Work out the finished part from the listing and answer in its coordinate system (mm). A direction names the side the tool comes from. Give positions to 0.01 mm unless a question says otherwise; leave off trailing zeros. Loops run counter-clockwise (first coordinate to the right, second up) from the corner with the lowest first, then second, coordinate; pieces in that order, holes last. Notation, with made-up numbers: M 87.5,71 L 145.5,71 A21 ccw 145.5,79 Z; hole C -0.5,-17 d4. An arc over 180 degrees is marked long. Answer as a JSON object with one key per item and string values. Group by question number.
```python
from build123d import *

# Parameters (mm, degrees)
SALIENTE_EXTRUIR1_DEPTH = 3
SALIENTE_EXTRUIR2_DEPTH = 9.75
CROQUIS6_R              = 1.625
CORTAR_EXTRUIR1_DEPTH   = 5
CORTAR_EXTRUIR2_DEPTH   = 2
CORTAR_EXTRUIR4_DEPTH   = 10
CROQUIS10_R             = 1.625
SALIENTE_EXTRUIR3_DEPTH = 2
CROQUIS12_R             = 1.625
CORTAR_EXTRUIR5_DEPTH   = 5
CORTAR_EXTRUIR6_DEPTH   = 2
CROQUIS14_R             = 1.625
CORTAR_EXTRUIR7_DEPTH   = 4
CORTAR_EXTRUIR8_DEPTH   = 2
CROQUIS17_R             = 1.625
CORTAR_EXTRUIR9_DEPTH   = 4
CORTAR_EXTRUIR10_DEPTH  = 2


with BuildPart() as part:
    # Croquis1 → Saliente-Extruir1 (new body)
    with BuildSketch(Plane.XY):
        with BuildLine():
            Line((0, 0.68070798), (0, 0))
            Line((0, 0), (72.78319995, 0))
            Line((72.78319995, 0), (55.699999998, 14.642073221))
            Line((55.699999998, 14.642073221), (46.67593732, 50.511923567))
            Line((46.67593732, 50.511923567), (-35.562657036, 50.511923567))
            Line((-35.562657036, 50.511923567), (-35.562657036, 38.25))
            Line((-35.562657036, 38.25), (-8.913300435, 38.25))
            Line((-8.913300435, 38.25), (-3.562657036, 35.25))
            ThreePointArc((-3.562657036, 35.25), (6.381456753, 18.806597842), (0, 0.68070798))
        make_face()
    extrude(amount=-SALIENTE_EXTRUIR1_DEPTH)

    # Croquis5 → Saliente-Extruir2 (add)
    with BuildSketch(Plane(origin=(0, 0, -3), x_dir=(-1, 0, 0), z_dir=(0, 0, -1))):
        with BuildLine():
            Line((-51.238983488, 11.880365447), (-59.266443595, 5))
            Line((-59.266443595, 5), (-3.339079606, 5))
            ThreePointArc((-3.339079606, 5), (-1.801031086, 2.738703104), (0, 0.68070798))
            Line((0, 0.68070798), (0, 0))
            Line((0, 0), (-72.78319995, 0))
            Line((-72.78319995, 0), (-55.699999998, 14.642073221))
            Line((-55.699999998, 14.642073221), (-46.67593732, 50.511923567))
            Line((-46.67593732, 50.511923567), (35.562657036, 50.511923567))
            Line((35.562657036, 50.511923567), (35.562657036, 38.25))
            Line((35.562657036, 38.25), (31.562657036, 38.25))
            Line((31.562657036, 38.25), (31.562657036, 46.511923567))
            Line((31.562657036, 46.511923567), (-42.526447804, 46.511923567))
            Line((-42.526447804, 46.511923567), (-51.238983488, 11.880365447))
        make_face()
    extrude(amount=SALIENTE_EXTRUIR2_DEPTH)

    # Croquis6 → Cortar-Extruir1 (cut)
    with BuildSketch(Plane.XZ):
        with Locations((6.999999998, -7)):
            Circle(CROQUIS6_R)
        with Locations((52.78319995, -7)):
            Circle(CROQUIS6_R)
    extrude(amount=-CORTAR_EXTRUIR1_DEPTH, mode=Mode.SUBTRACT)

    # Croquis8 → Cortar-Extruir2 (cut)
    with BuildSketch(Plane(origin=(0, 5, 0), x_dir=(1, 0, 0), z_dir=(0, 1, 0))):
        Polygon((3.819999998, 7), (5.409999998, 4.246039216), (8.589999998, 4.246039216), (10.179999998, 7), (8.589999998, 9.753960784), (5.409999998, 9.753960784), align=None)
        Polygon((49.60319995, 7), (51.19319995, 4.246039216), (54.37319995, 4.246039216), (55.96319995, 7), (54.37319995, 9.753960784), (51.19319995, 9.753960784), align=None)
    extrude(amount=-CORTAR_EXTRUIR2_DEPTH, mode=Mode.SUBTRACT)

    # Croquis9 → Cortar-Extruir4 (cut)
    with BuildSketch(Plane(origin=(30.824200619, 35.963211942, 0), x_dir=(0.759271307, -0.650774217, 0), z_dir=(0.650774217, 0.759271307, 0))):
        Polygon((50.442195378, 6.375), (48.852195378, 9.128960784), (45.672195378, 9.128960784), (44.082195378, 6.375), (45.672195378, 3.621039216), (48.852195378, 3.621039216), align=None)
    extrude(amount=-CORTAR_EXTRUIR4_DEPTH, mode=Mode.SUBTRACT)

    # Croquis10 → Saliente-Extruir3 (add)
    with BuildSketch(Plane(origin=(30.824200619, 35.963211942, 0), x_dir=(0.759271307, -0.650774217, 0), z_dir=(0.650774217, 0.759271307, 0))):
        Polygon((50.442195378, 6.375), (48.852195378, 9.128960784), (45.672195378, 9.128960784), (44.082195378, 6.375), (45.672195378, 3.621039216), (48.852195378, 3.621039216), align=None)
        with Locations((47.262195378, 6.375)):
            Circle(CROQUIS10_R, mode=Mode.SUBTRACT)
    extrude(amount=-SALIENTE_EXTRUIR3_DEPTH)

    # Croquis12 → Cortar-Extruir5 (cut)
    with BuildSketch(Plane(origin=(55.848866467, 14.050342186, 0), x_dir=(0, 0, -1), z_dir=(0.969781373, 0.24397559, 0))):
        with Locations((6.375, 23.727396855)):
            Circle(CROQUIS12_R)
    extrude(amount=-CORTAR_EXTRUIR5_DEPTH, mode=Mode.SUBTRACT)

    # Croquis13 → Cortar-Extruir6 (cut)
    with BuildSketch(Plane(origin=(50.999959602, 12.830464236, 0), x_dir=(0, 0, 1), z_dir=(-0.969781373, -0.24397559, 0))):
        Polygon((-6.375, 20.547396855), (-3.621039216, 22.137396855), (-3.621039216, 25.317396855), (-6.375, 26.907396855), (-9.128960784, 25.317396855), (-9.128960784, 22.137396855), align=None)
    extrude(amount=-CORTAR_EXTRUIR6_DEPTH, mode=Mode.SUBTRACT)

    # Croquis14 → Cortar-Extruir7 (cut)
    with BuildSketch(Plane(origin=(0, 50.511923567, 0), x_dir=(1, 0, 0), z_dir=(0, 1, 0))):
        with Locations((-25.562657036, 6.375)):
            Circle(CROQUIS14_R)
        with Locations((24.437342964, 6.375)):
            Circle(CROQUIS14_R)
    extrude(amount=-CORTAR_EXTRUIR7_DEPTH, mode=Mode.SUBTRACT)

    # Croquis15 → Cortar-Extruir8 (cut)
    with BuildSketch(Plane.XZ.offset(-46.511923567)):
        Polygon((-22.382657036, -6.375), (-23.972657036, -3.621039216), (-27.152657036, -3.621039216), (-28.742657036, -6.375), (-27.152657036, -9.128960784), (-23.972657036, -9.128960784), align=None)
        Polygon((21.257342964, -6.375), (22.847342964, -9.128960784), (26.027342964, -9.128960784), (27.617342964, -6.375), (26.027342964, -3.621039216), (22.847342964, -3.621039216), align=None)
    extrude(amount=-CORTAR_EXTRUIR8_DEPTH, mode=Mode.SUBTRACT)

    # Croquis17 → Cortar-Extruir9 (cut)
    with BuildSketch(Plane.ZY.offset(35.562657036)):
        with Locations((-7.982505966, 42.38)):
            Circle(CROQUIS17_R)
    extrude(amount=-CORTAR_EXTRUIR9_DEPTH, mode=Mode.SUBTRACT)

    # Croquis18 → Cortar-Extruir10 (cut)
    with BuildSketch(Plane(origin=(-31.562657036, 0, 0), x_dir=(0, 0, -1), z_dir=(1, 0, 0))):
        Polygon((7.982505966, 39.2), (10.73646675, 40.79), (10.73646675, 43.97), (7.982505966, 45.56), (5.228545182, 43.97), (5.228545182, 40.79), align=None)
    extrude(amount=-CORTAR_EXTRUIR10_DEPTH, mode=Mode.SUBTRACT)


solid = part.part
```
Item 1: For a pull along Z with two mould halves and no side action, classify faces 5 (the flat face through (-6.275, 36.771, -1.479)), 6 (the flat face through (66.34, 1.13, -4.98)), 7 (the flat face through (18, 26, 0)) as pulls with the +Z half, pulls with the -Z half, needs draft (parallel to the pull), parting line crosses it, or undercut.
Item 2: A tool of negligible diameter and unlimited length cuts with its end or side. For faces 1 (the flat face through (5, 46.512, -8)), 2 (the cylindrical face through (-34.577, 40.794, -8.335)), 3 (the flat face through (55.18, 4.01, -8.36)), 4 (the flat face through (-26, 47, -3.621)), from which of +Z, -Z, +X, -X, +Y, -Y can it reach the whole face along a straight path? Write none if from no direction.
Item 3: Given pin 1 Ø5 at (y, z) = (25.5, -2.5) entering from -X; pin 2 Ø0.6 at (x, y) = (-25.5, 47.5) entering from +Z; pin 3 Ø3 at (y, z) = (35, -6.5) entering from -X; pin 4 Ø2 at (y, z) = (6.5, -2) entering from +X, each flat-ended and moving along its own axis, determine where each tip first touches the part or whether it passes through.
Item 4: A cutting plane is placed at D-D (y = 31.5). Determine the outline of the cut face in (x, z).
Item 5: Find the intervals of material crossed by probe 1 along Y at (x, z) = (32, -9.75); probe 2 along Z at (x, y) = (-30, 40); probe 3 along Z at (x, y) = (7, 1) (3 decimals), in increasing order. Write a range as [from, to].
Item 6: A cutting plane is placed at B-B (x = 14). Determine the outline of the cut face in (y, z), and give its area (3 significant figures).
Item 7: A cutting plane is placed at A-A (y = 42.38). Determine the outline of the cut face in (x, z).
Item 8: A cutting plane is placed at C-C (z = -1.75). Determine the outline of the cut face in (x, y), and give its area (3 significant figures).
The answers:
{
 "1": {"face 5": "needs draft", "face 6": "undercut", "face 7": "pulls with the +Z half"},
 "2": {"face 1": "-Z", "face 2": "-X", "face 3": "none", "face 4": "-Y"},
 "3": {"pin 1": "stops at x = 3.34", "pin 2": "stops at z = 0", "pin 3": "stops at x = 47.32", "pin 4": "stops at x = 66.37"},
 "4": {"outline": "M 0.77,-3 L 46.3,-3 L 46.3,-12.75 L 51.46,-12.75 L 51.46,0 L 0.77,0 Z"},
 "5": {"probe 1": "y = [0, 5], [46.51, 50.51]", "probe 2": "z = [-3, 0]", "probe 3": "z = [-12.75, -8.625], [-5.375, 0]"},
 "6": {"outline": "M 0,-12.75 L 5,-12.75 L 5,-3 L 46.51,-3 L 46.51,-12.75 L 50.51,-12.75 L 50.51,0 L 0,0 Z", "area": "239 mm^2"},
 "7": {"outline": "M -35.56,-12.75 L -31.56,-12.75 L -31.56,-10.74 L -33.56,-10.74 L -33.56,-9.61 L -35.56,-9.61 Z; M -35.56,-6.36 L -33.56,-6.36 L -33.56,-5.23 L -31.56,-5.23 L -31.56,-3 L 43.57,-3 L 43.57,-12.75 L 48.72,-12.75 L 48.72,0 L -35.56,0 Z"},
 "8": {"outline": "M -35.56,38.25 L -8.91,38.25 L -3.56,35.25 A22.5 cw 0,0.68 L 0,0 L 72.78,0 L 55.7,14.64 L 46.68,50.51 L -35.56,50.51 Z", "area": "3,090 mm^2"}
}
